The model under review builds one solid part; all positions refer to its coordinate system, in mm. A direction names the side the tool comes from. Round coordinates to 2 decimals unless told otherwise and drop trailing zeros. Write each loop counter-clockwise with the first axis right and the second up, starting at its lowest first coordinate (ties: lowest second). Pieces come first, ordered by that corner, then holes. Notation, with made-up numbers: (68, 69.5) - (82, 69.5) arc R11 cw to (82, 81.5) - close; hole circle Ø4 at (-16.5, 75.25). An arc over 180 degrees is marked (long way). Return JSON: item names as keys, results as strings.
from build123d import *

# Parameters (mm, degrees)
SKETCH_1_R          = 0.5
EXTRUDE_1_DEPTH     = 2
SKETCH_2_R          = 4.5
SKETCH_2_R_2        = 2.5
EXTRUDE_2_DEPTH     = 5
SKETCH_3_R          = 3.5
CUT_EXTRUDE_1_DEPTH = 4
SKETCH_5_R          = 1.5
CUT_EXTRUDE_2_DEPTH = 10


with BuildPart() as part:
    # 草图1 → 凸台-拉伸1 (new body)
    with BuildSketch(Plane.XY):
        with BuildLine():
            Line((16.5, -3.799671038), (4.823155871, -5.182135299))
            ThreePointArc((4.823155871, -5.182135299), (3.914969309, -5.376520098), (3.058401724, -5.735519061))
            ThreePointArc((3.058401724, -5.735519061), (0, -6.5), (-3.058401724, -5.735519061))
            ThreePointArc((-3.058401724, -5.735519061), (-3.914969309, -5.376520098), (-4.823155871, -5.182135299))
            Line((-4.823155871, -5.182135299), (-16.5, -3.799671038))
            ThreePointArc((-16.5, -3.799671038), (-19.25, 0), (-16.5, 3.799671038))
            Line((-16.5, 3.799671038), (-4.823155871, 5.182135299))
            ThreePointArc((-4.823155871, 5.182135299), (-3.914969309, 5.376520098), (-3.058401724, 5.735519061))
            ThreePointArc((-3.058401724, 5.735519061), (0, 6.5), (3.058401724, 5.735519061))
            ThreePointArc((3.058401724, 5.735519061), (3.914969309, 5.376520098), (4.823155871, 5.182135299))
            Line((4.823155871, 5.182135299), (16.5, 3.799671038))
            ThreePointArc((16.5, 3.799671038), (19.25, 0), (16.5, -3.799671038))
        make_face()
        with Locations((-16.5, 0)):
            Circle(SKETCH_1_R, mode=Mode.SUBTRACT)
        with Locations((-12.75, 0)):
            Circle(SKETCH_1_R, mode=Mode.SUBTRACT)
        with Locations((-9.75, 0)):
            Circle(SKETCH_1_R, mode=Mode.SUBTRACT)
        with Locations((-6.75, 0)):
            Circle(SKETCH_1_R, mode=Mode.SUBTRACT)
        with Locations((-3.75, 0)):
            Circle(SKETCH_1_R, mode=Mode.SUBTRACT)
        with Locations(Location((3.75, 0, 0), (0, 0, 180))):
            Circle(SKETCH_1_R, mode=Mode.SUBTRACT)
        with Locations(Location((6.75, 0, 0), (0, 0, 180))):
            Circle(SKETCH_1_R, mode=Mode.SUBTRACT)
        with Locations(Location((9.75, 0, 0), (0, 0, 180))):
            Circle(SKETCH_1_R, mode=Mode.SUBTRACT)
        with Locations(Location((12.75, 0, 0), (0, 0, 180))):
            Circle(SKETCH_1_R, mode=Mode.SUBTRACT)
        with Locations(Location((16.5, 0, 0), (0, 0, 180))):
            Circle(SKETCH_1_R, mode=Mode.SUBTRACT)
    extrude(amount=EXTRUDE_1_DEPTH)

    # 草图2 → 凸台-拉伸2 (add)
    with BuildSketch(Plane.XY.offset(2)):
        Circle(SKETCH_2_R)
        Circle(SKETCH_2_R_2, mode=Mode.SUBTRACT)
    extrude(amount=EXTRUDE_2_DEPTH)

    # 草图3 → 切除-拉伸1 (cut)
    with BuildSketch(Plane(origin=(0, 0, 0), x_dir=(-1, 0, 0), z_dir=(0, 0, -1))):
        Circle(SKETCH_3_R)
    extrude(amount=-CUT_EXTRUDE_1_DEPTH, mode=Mode.SUBTRACT)

    # 草图5 → 切除-拉伸2 (cut)
    with BuildSketch(Plane.XY.offset(2)):
        with Locations((16.5, 0)):
            Circle(SKETCH_5_R)
        with Locations((-16.5, 0)):
            Circle(SKETCH_5_R)
    extrude(amount=-CUT_EXTRUDE_2_DEPTH, mode=Mode.SUBTRACT)


solid = part.part
(1) Add section C-C (y = -3). Write out the cut boundary in (x, z), plus the area to 3 significant figures.
Filled in:
{"outline": "(-17.9, 0) - (-1.8, 0) - (-1.8, 4) - (1.8, 4) - (1.8, 0) - (17.9, 0) - (17.9, 2) - (3.35, 2) - (3.35, 7) - (-3.35, 7) - (-3.35, 2) - (-17.9, 2) - close", "area": "90.7 mm2"}
(2) Add section A-A (x = 0). Write out the cut boundary in (y, z), plus the area to 3 significant figures.
Filled in:
{"outline": "(-6.5, 0) - (-3.5, 0) - (-3.5, 4) - (-2.5, 4) - (-2.5, 7) - (-4.5, 7) - (-4.5, 2) - (-6.5, 2) - close; (2.5, 4) - (3.5, 4) - (3.5, 0) - (6.5, 0) - (6.5, 2) - (4.5, 2) - (4.5, 7) - (2.5, 7) - close", "area": "28.0 mm2"}
(3) Add section D-D (y = 0). Give the number of separate pieces and of enclosed holes in the cut face, plus the area to 3 significant figures.
Filled in:
{"separate pieces": "10", "enclosed holes": "0", "area": "52.0 mm2"}
(4) For faces 5 (the cylindrical face through (3.93, -5.37, 0.99)), 6 (the cylindrical face through (-4.25, 0.02, 0.99)), list the 3-axis set-ups (+Z, -Z, +X, -X, +Y, -Y) from which the entire face can be reached by the end or side of a thin tool; tool diameter is ignored.
Filled in:
{"face 5": "+Z, -Z, +X, -Y", "face 6": "-Z"}
(5) Wall thickness on line 1 (Y direction, x = 0, z = 3.5); line 2 (Y direction, x = -16.5, z = 1.05); line 3 (Z direction, x = 9, y = 4): over which ranges is each line inside the solid? List them lowest first.
Filled in:
{"line 1": "y = -4.5 to -3.5, 3.5 to 4.5", "line 2": "y = -3.8 to -1.5, 1.5 to 3.8", "line 3": "z = 0 to 2"}
(6) Add section B-B (z = 2.5). Write out the cut boundary in (x, y).
Filled in:
{"outline": "circle Ø9 at (0, 0); hole circle Ø7 at (0, 0)"}
(7) Clearance check with flat-ended pins moving along their axes: pin 1 Ø6.5 at (x, y) = (0, 0) entering from -Z; pin 2 Ø6.5 at (x, y) = (7.5, -1.5) entering from +Z; pin 3 Ø3.5 at (x, y) = (-16.5, 0) entering from +Z. State where each tip first meets the part, or that it passes through.
Filled in:
{"pin 1": "stops at z = 4", "pin 2": "stops at z = 7", "pin 3": "stops at z = 2"}
(8) Mouldability with a two-part tool opening along Y and no side actions: class faces 1 (the cylindrical face through (10.25, -0.02, 0.99)), 2 (the flat face through (-10.6, -4.5, 1)), 3 (the cylindrical face through (4.25, -0.02, 0.99)), 4 (the cylindrical face through (19.25, 0.07, 0.99)) as released by +Y, released by -Y, zero draft, split by the parting line, or undercut.
Filled in:
{"face 1": "undercut", "face 2": "released by -Y", "face 3": "undercut", "face 4": "split by the parting line"}
